Design review of the part built by this model. Coordinates are the model's own, in mm. A direction names the side the tool comes from. Coordinates: 2 decimals unless noted, no trailing zeros. Write each loop counter-clockwise with the first axis right and the second up, starting at its lowest first coordinate (ties: lowest second). Pieces come first, ordered by that corner, then holes. Notation, with made-up numbers: M -30,81 L -10,81 A14 cw -10,92 Z; hole C -1,85 d5. An arc over 180 degrees is marked long. Write each question's results on one line, items separated by ' | '. Start each with the question number.
Autodesk Inventor part; units mm, degrees
ref_plane "Work Plane1" through (-13.2447, 0, 62.195) normal (1, 0, 0) x (0, 1, 0)
ref_plane "XZ Plane" through (0, 0, 0) normal (0, 1, 0) x (-1, 0, 0)
ref_plane "XY Plane" through (0, 0, 0) normal (0, 0, 1) x (1, 0, 0)
sketch "Sketch2" plane through (0, 0, 0) normal (0, 1, 0) x (-1, 0, 0)
  line L0 (0, 0) -> (0, 80)
  line L1 (0, 80) -> (-13.2447, 80)
  line L2 (-13.2447, 80) -> (-13.2447, 44.3901)
  line L3 (-22.5598, 44.3901) -> (-22.5598, 31.5867)
  line L4 (-22.5598, 31.5867) -> (-15, 31.5867)
  line L5 (-15, 31.5867) -> (-15, 0)
  line L6 (-15, 0) -> (0, 0)
  line L7 (-22.5598, 44.3901) -> (-13.2447, 44.3901)
  dimension "d6" = 30
  dimension "d7" = 80
revolve "Revolution1" add sketch "Sketch2" angle 360 about axis through (0, 0, 0) along (0, 0, 1)
ref_plane "Work Plane1" through (-13.2447, 0, 62.195) normal (1, 0, 0) x (0, 1, 0)
sketch "Sketch3" plane through (-13.2447, 0, 62.195) normal (1, 0, 0) x (0, 1, 0)
  line L0 (13.2447, -17.805) -> (-13.2447, -17.805)
  line L1 (13.2447, 17.805) -> (-13.2447, 17.805)
  line L2 (0.1403, 5.805) -> (0.1403, -4.195) construction
  line L3 (-3.8597, 5.805) -> (-3.8597, -4.195)
  line L4 (4.1403, -4.195) -> (4.1403, 5.805)
  arc A0 (4.1403, 5.805) -> (-3.8597, 5.805) centre (0.1403, 5.805) ccw
  arc A1 (-3.8597, -4.195) -> (4.1403, -4.195) centre (0.1403, -4.195) ccw
  point P0 (0, -62.195)
  point P1 (0.1403, 0.805)
  dimension "d8" = 12
  dimension "d9" = 8
  dimension "d10" = 10
extrude "Extrusion2" cut sketch "Sketch3" along normal blind 10
properties part number "NVPH-312 augur shaft"
Item 1: We need section C-C on y = 7. State the section outline as (x, z) points.
Item 2: Insertion check: pin 1 Ø2 at (x, y) = (9, -13) entering from +Z; pin 2 Ø8 at (x, y) = (11.5, -16.5) entering from -Z; pin 3 Ø5 at (y, z) = (12.5, 11) entering from +X. Each pin has a flat end and moves straight along its axis. Give the tip position at first contact, or say it passes through.
Item 3: We need section A-A on x = 0. State the section outline as (y, z) points, then the cut area to 3 significant figures.
Item 4: We need section B-B on x = -11. State the section outline as (y, z) points.
Item 5: We need section D-D on z = 23.5. State the section outline as (x, y) points, then the cut area to 3 significant figures.
Item 6: Draft analysis for pull direction Y (two halves, no side actions). For faces 1 (the flat face through (15, -5, 31.587)), 2 (the cylindrical face through (-8.3, 0.1, 72)), 3 (the cylindrical face through (12.633, -3.978, 61.946)), state which applies: released by +Y, released by -Y, zero draft, split by the parting line, or undercut.
Item 7: Wall thickness on L1, parallel to X at y = 0, z = 71; L2, parallel to Z at x = -6.5, y = -12; L3, parallel to Y at x = 9, z = 65: over which ranges is each line inside the solid? List them lowest first.
Item 8: For faces 4 (the flat face through (-3.245, 0, 63)), 5 (the cylindrical face through (-14.985, -0.66, 15.572)), 6 (the flat face through (10, -10, 44.39)), 7 (the flat face through (0, 0, 0)), list the 3-axis set-ups (+Z, -Z, +X, -X, +Y, -Y) from which the entire face can be reached by the end or side of a thin tool; tool diameter is ignored.
Answer:
1) outline: M -21.45,31.59 L -13.27,31.59 L -13.27,0 L 13.27,0 L 13.27,31.59 L 21.45,31.59 L 21.45,44.39 L 11.24,44.39 L 11.24,80 L -11.24,80 L -11.24,44.39 L -21.45,44.39 Z
2) pin 1: stops at z = 44.39 | pin 2: stops at z = 31.59 | pin 3: stops at x = 11.18
3) outline: M -22.56,31.59 L -15,31.59 L -15,0 L 15,0 L 15,31.59 L 22.56,31.59 L 22.56,44.39 L 13.24,44.39 L 13.24,80 L -13.24,80 L -13.24,44.39 L -22.56,44.39 Z | area: 2,470 mm^2
4) outline: M -19.7,31.59 L -10.2,31.59 L -10.2,0 L 10.2,0 L 10.2,31.59 L 19.7,31.59 L 19.7,44.39 L 7.38,44.39 L 7.38,80 L -7.38,80 L -7.38,44.39 L -19.7,44.39 Z; hole M -3.86,58 A4 ccw 4.14,58 L 4.14,68 A4 ccw -3.86,68 Z
5) outline: C 0,0 d30 | area: 707 mm^2
6) face 1: zero draft | face 2: undercut | face 3: split by the parting line
7) L1: x = -3.24 to 13.24 | L2: z = 0 to 44.39 | L3: y = -9.72 to 9.72
8) face 4: -X | face 5: -Z | face 6: +Z | face 7: -Z, +X, -X, +Y, -Y
